```python
from build123d import *

# Parameters (mm, degrees)
F0_W     = 50.8
F0_H     = 50.8
F1_DEPTH = 50.8
F2_R     = 13.262448
F3_DEPTH = 50.801
F4_R     = 5.08
F5_R     = 2.8575
F6_DEPTH = 50.801


with BuildPart() as f1:
    # F0 (on Top) → F1 (new body)
    with BuildSketch(Plane.XY):
        with Locations((25.4, 25.4)):
            Rectangle(F0_W, F0_H)
    extrude(amount=F1_DEPTH)

    # F2 (on face) → F3 (cut, through all)
    with BuildSketch(Plane.YZ.offset(50.8)):
        with Locations((25.4, 25.4)):
            Circle(F2_R)
    extrude(amount=-F3_DEPTH, mode=Mode.SUBTRACT)

    # F4
    f4_edges = [f1.edges().sort_by_distance(p)[0] for p in [
        (25.4, 50.8, 50.8),
        (25.4, 0, 50.8),
        (25.4, 50.8, 0),
        (25.4, 0, 0),
    ]]
    fillet(f4_edges, radius=F4_R)

    # F5 (on face) → F6 (cut, through all)
    with BuildSketch(Plane.YZ.offset(50.8)):
        with Locations((43.18, 43.18)):
            Circle(F5_R)
    extrude(amount=-F6_DEPTH, mode=Mode.SUBTRACT)


solid = f1.part
```
Input: part model. Units: mm. Frame: model coordinates. Coordinates: 2 decimals unless noted, no trailing zeros. Loops run counter-clockwise (first coordinate to the right, second up) from the corner with the lowest first, then second, coordinate; pieces in that order, holes last. Notation, with made-up numbers: M 69,18 L 128,18 A24 ccw 128,31 Z; hole C 29,57.25 d11. An arc over 180 degrees is marked long. One line per item, written item: value.
(1) Pin query (flat end, axial travel): pin 1 (5 mm diameter, centred on y = 43.18, z = 43.18, fed in from -X). Return the tip coordinate at first contact, or that it passes through.
Filled in:
pin 1: through
(2) Section A-A (z = 25.4). Output: boundary loops of the cut face in (x, y), and give its area (3 significant figures).
Filled in:
outline: M 0,0 L 50.8,0 L 50.8,12.14 L 0,12.14 Z; M 0,38.66 L 50.8,38.66 L 50.8,50.8 L 0,50.8 Z
area: 1,230 mm^2
(3) Line query: line 1 along Z through (x, y) = (9, 43); line 2 along Y through (x, z) = (35, 25). Output: solid intervals per line, ascending. Write a range as from..to.
Filled in:
line 1: 0..40.33, 46.03..50.8
line 2: 0..12.14, 38.66..50.8
(4) Section C-C (x = 25). Output: boundary loops of the cut face in (y, z) (1 decimal), and give its area (3 significant figures).
Filled in:
outline: M 0,5.1 A5.1 ccw 5.1,0 L 45.7,0 A5.1 ccw 50.8,5.1 L 50.8,45.7 A5.1 ccw 45.7,50.8 L 5.1,50.8 A5.1 ccw 0,45.7 Z; hole C 25.4,25.4 d26.5; hole C 43.2,43.2 d5.7
area: 1,980 mm^2
(5) Section B-B (y = 43.18). Output: boundary loops of the cut face in (x, z), and give its area (3 significant figures).
Filled in:
outline: M 0,0 L 50.8,0 L 50.8,40.32 L 0,40.32 Z; M 0,46.04 L 50.8,46.04 L 50.8,50.8 L 0,50.8 Z
area: 2,290 mm^2
(6) Pull-direction query (Y, two-part tool) for faces 1 (the cylindrical face through (25.756, 1.449, 49.272)), 2 (the cylindrical face through (25.756, 49.272, 49.351)), 3 (the cylindrical face through (25.756, 40.325, 43.306)), 4 (the cylindrical face through (25.756, 22.525, 12.453)); classes: +Y half, -Y half, draft (parallel to the pull), parting line (faces both ways), or undercut.
Filled in:
face 1: -Y half
face 2: +Y half
face 3: undercut
face 4: undercut
